Verification items for the finished model (mm, model axes). Face numbers are marked on the shaded views. A direction names the side the tool comes from. Coordinates: 2 decimals unless noted, no trailing zeros. Loops run counter-clockwise (first coordinate to the right, second up) from the corner with the lowest first, then second, coordinate; pieces in that order, holes last. Notation, with made-up numbers: (65.5, 9) -> (121.5, 9) arc R22 ccw to (121.5, 38) -> close; hole circle Ø8 at (66.25, 53). An arc over 180 degrees is marked (long way). Write item = value, one per line.
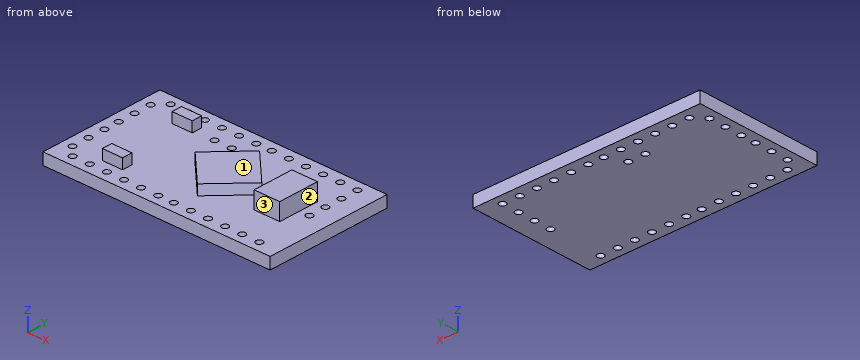
```python
from build123d import *

# Parameters (mm, degrees)
F0_W     = 33.7
F0_H     = 18.6
F1_DEPTH = 1.7
F2_R     = 0.5
F3_DEPTH = 1.701
F5_DEPTH = 1.5
F4_W     = 3.8
F4_H     = 6
F6_DEPTH = 2.5
F4_W_2   = 3
F4_H_2   = 1.5
F7_DEPTH = 1.5


with BuildPart() as f1:
    # F0 (on Top) → F1 (new body)
    with BuildSketch(Plane.XY):
        Rectangle(F0_W, F0_H)
    extrude(amount=F1_DEPTH)

    # F2 (on face) → F3 (cut, through all)
    with BuildSketch(Plane.XY.offset(1.7)):
        with Locations((-13.85, 7.8)):
            Circle(F2_R)
        with Locations((-11.31, 7.8)):
            Circle(F2_R)
        with Locations((-8.77, 7.8)):
            Circle(F2_R)
        with Locations((-6.23, 7.8)):
            Circle(F2_R)
        with Locations((-3.69, 7.8)):
            Circle(F2_R)
        with Locations((-1.15, 7.8)):
            Circle(F2_R)
        with Locations((1.15, 7.8)):
            Circle(F2_R)
        with Locations((3.69, 7.8)):
            Circle(F2_R)
        with Locations((6.23, 7.8)):
            Circle(F2_R)
        with Locations((8.77, 7.8)):
            Circle(F2_R)
        with Locations((11.31, 7.8)):
            Circle(F2_R)
        with Locations((13.85, 7.8)):
            Circle(F2_R)
        with Locations((13.85, -7.8)):
            Circle(F2_R)
        with Locations((11.31, -7.8)):
            Circle(F2_R)
        with Locations((8.77, -7.8)):
            Circle(F2_R)
        with Locations((6.23, -7.8)):
            Circle(F2_R)
        with Locations((3.69, -7.8)):
            Circle(F2_R)
        with Locations((1.15, -7.8)):
            Circle(F2_R)
        with Locations((-1.15, -7.8)):
            Circle(F2_R)
        with Locations((-3.69, -7.8)):
            Circle(F2_R)
        with Locations((-6.23, -7.8)):
            Circle(F2_R)
        with Locations((-8.77, -7.8)):
            Circle(F2_R)
        with Locations((-11.31, -7.8)):
            Circle(F2_R)
        with Locations((-13.85, -7.8)):
            Circle(F2_R)
        with Locations((13.85, 5.26)):
            Circle(F2_R)
        with Locations((13.85, 2.72)):
            Circle(F2_R)
        with Locations((13.85, 0.18)):
            Circle(F2_R)
        with Locations((-15.35, 6.215414)):
            Circle(F2_R)
        with Locations((-15.35, 3.675414)):
            Circle(F2_R)
        with Locations((-15.35, 1.135414)):
            Circle(F2_R)
        with Locations((-15.35, -1.135414)):
            Circle(F2_R)
        with Locations((-15.35, -3.675414)):
            Circle(F2_R)
        with Locations((-15.35, -6.215414)):
            Circle(F2_R)
        with Locations((-4.96, 5.26)):
            Circle(F2_R)
        with Locations((-2.42, 5.26)):
            Circle(F2_R)
    extrude(amount=-F3_DEPTH, mode=Mode.SUBTRACT)

    # F4 (on face) → F5 (join)
    with BuildSketch(Plane.XY.offset(1.7)):
        Polygon((6.949747, 0), (2, 4.949747), (-2.949747, 0), (2, -4.949747), align=None)
    extrude(amount=F5_DEPTH)

    # F4 (on face) → F6 (join)
    with BuildSketch(Plane.XY.offset(1.7)):
        with Locations((10.5, 0)):
            Rectangle(F4_W, F4_H)
    extrude(amount=F6_DEPTH)

    # F4 (on face) → F7 (join)
    with BuildSketch(Plane.XY.offset(1.7)):
        with Locations((-9.35, 5.55)):
            Rectangle(F4_W_2, F4_H_2)
        with Locations((-9.35, -5.55)):
            Rectangle(F4_W_2, F4_H_2)
    extrude(amount=F7_DEPTH)


solid = f1.part
```
1) Sectioned sample at B-B, the plane x = -2.42. Record the cut outline in (y, z).
Ans:
outline = (-9.3, 0) -> (4.76, 0) -> (4.76, 1.7) -> (0.53, 1.7) -> (0.53, 3.2) -> (-0.53, 3.2) -> (-0.53, 1.7) -> (-9.3, 1.7) -> close; (5.76, 0) -> (9.3, 0) -> (9.3, 1.7) -> (5.76, 1.7) -> close
2) Tool access check on the marked faces 1, 2 and 3. Record the directions out of +Z, -Z, +X, -X, +Y, -Y that give a thin tool (end or side, any length) a straight path to the whole face; none if there is none.
Ans:
face_1 = +Z, -X, +Y, -Y
face_2 = +Z, +X, +Y, -Y
face_3 = +Z, +X, -Y
3) Depth check by flat-ended pin: pin 1 Ø1 at (x, z) = (7, 3) entering from +Y; pin 2 Ø1.6 at (y, z) = (-5.5, 2) entering from -X; pin 3 Ø2 at (y, z) = (-0.5, 3.5) entering from +X; pin 4 Ø0.8 at (x, z) = (-9.5, 2.5) entering from -Y. Enter the tip coordinate at first touch or a pass-through.
Ans:
pin_1 = 0.45
pin_2 = -16.85
pin_3 = 12.4
pin_4 = -6.3
4) Sectioned sample at A-A, the plane z = 2.1. Record the cut outline in (x, y), plus the area to 3 significant figures.
Ans:
outline = (-10.85, -6.3) -> (-7.85, -6.3) -> (-7.85, -4.8) -> (-10.85, -4.8) -> close; (-10.85, 4.8) -> (-7.85, 4.8) -> (-7.85, 6.3) -> (-10.85, 6.3) -> close; (-2.95, 0) -> (2, -4.95) -> (6.95, 0) -> (2, 4.95) -> close; (8.6, -3) -> (12.4, -3) -> (12.4, 3) -> (8.6, 3) -> close
area = 80.8 mm2
5) Sectioned sample at D-D, the plane x = 6.23. Record the cut outline in (y, z).
Ans:
outline = (-9.3, 0) -> (-8.3, 0) -> (-8.3, 1.7) -> (-9.3, 1.7) -> close; (-7.3, 0) -> (7.3, 0) -> (7.3, 1.7) -> (0.72, 1.7) -> (0.72, 3.2) -> (-0.72, 3.2) -> (-0.72, 1.7) -> (-7.3, 1.7) -> close; (8.3, 0) -> (9.3, 0) -> (9.3, 1.7) -> (8.3, 1.7) -> close
6) Sectioned sample at C-C, the plane x = 1.15. Record the cut outline in (y, z), plus the area to 3 significant figures.
Ans:
outline = (-9.3, 0) -> (-8.3, 0) -> (-8.3, 1.7) -> (-9.3, 1.7) -> close; (-7.3, 0) -> (7.3, 0) -> (7.3, 1.7) -> (4.1, 1.7) -> (4.1, 3.2) -> (-4.1, 3.2) -> (-4.1, 1.7) -> (-7.3, 1.7) -> close; (8.3, 0) -> (9.3, 0) -> (9.3, 1.7) -> (8.3, 1.7) -> close
area = 40.5 mm2
7) Material ranges on line 1 (Y direction, x = 6.23, z = 0.75); line 2 (Z direction, x = -13, y = -1.5); line 3 (X direction, y = -2.5, z = 3.05), recorded low to high.
Ans:
line_1 = -9.3 to -8.3, -7.3 to 7.3, 8.3 to 9.3
line_2 = 0 to 1.7
line_3 = -0.45 to 4.45, 8.6 to 12.4
